Solid Edge part; units mm, degrees
sketch "Sketch1" plane through (0, 0, 0) normal (0, 0, 1) x (1, 0, 0)
  arc A0 (-2.2, 0) -> (-0.6464, 2.8) centre (1.1, 0) cw
  line L0 (-0.6464, 2.8) -> (0, 2.8)
  line L1 (0, 2.8) -> (0, 1.55)
  arc A1 (0, 1.55) -> (0.1, 1.45) centre (0.1, 1.55) ccw
  line L2 (0.1, 1.45) -> (3.9885, 1.45)
  line L3 (3.9885, 1.45) -> (6.5, 0)
  line L4 (6.5, 0) -> (-2.2, 0)
revolve "RevolvedProtrusion1" add sketch "Sketch1" angle 360 about axis through (6.5, 0, 0) along (-1, 0, 0)
sketch "Sketch2" plane through (-2.2, 0, 0) normal (1, 0, 0) x (0, 1, 0)
  line L0 (0.2375, 0.95) -> (-0.2375, 0.95)
  line L1 (-0.2375, 0.95) -> (-0.66, 0.66)
  line L2 (-0.66, 0.66) -> (-0.95, 0.2375)
  line L3 (-0.95, 0.2375) -> (-0.95, -0.2375)
  line L4 (-0.95, -0.2375) -> (-0.66, -0.66)
  line L5 (-0.66, -0.66) -> (-0.2375, -0.95)
  line L6 (-0.2375, -0.95) -> (0.2375, -0.95)
  line L7 (0.2375, -0.95) -> (0.66, -0.66)
  line L8 (0.66, -0.66) -> (0.95, -0.2375)
  line L9 (0.95, -0.2375) -> (0.95, 0.2375)
  line L10 (0.95, 0.2375) -> (0.66, 0.66)
  line L11 (0.66, 0.66) -> (0.2375, 0.95)
extrude "ExtrudedCutout_1" cut sketch "Sketch2" along normal blind 0.7333
sketch "Sketch3" plane through (-2.2, 0, 0) normal (1, 0, 0) x (0, 1, 0)
  line L0 (0.1187, 0.475) -> (-0.1187, 0.475)
  line L1 (-0.1187, 0.475) -> (-0.33, 0.33)
  line L2 (-0.33, 0.33) -> (-0.475, 0.1188)
  line L3 (-0.475, 0.1188) -> (-0.475, -0.1187)
  line L4 (-0.475, -0.1187) -> (-0.33, -0.33)
  line L5 (-0.33, -0.33) -> (-0.1187, -0.475)
  line L6 (-0.1187, -0.475) -> (0.1187, -0.475)
  line L7 (0.1187, -0.475) -> (0.33, -0.33)
  line L8 (0.33, -0.33) -> (0.475, -0.1187)
  line L9 (0.475, -0.1187) -> (0.475, 0.1188)
  line L10 (0.475, 0.1188) -> (0.33, 0.33)
  line L11 (0.33, 0.33) -> (0.1187, 0.475)
extrude "ExtrudedCutout_2" cut sketch "Sketch3" along normal blind 0.88
properties part number "bene_inox_212406-2,9X6,5"
Can you work these out from the model? Positions are in its coordinate system, mm. Give positions to 0.01 mm unless a question says otherwise; leave off trailing zeros. Order: outer loops, then holes, each group sorted by start corner. A loop starts at its lowest first (then second) coordinate and runs counter-clockwise, first axis right, second up. Notation, with made-up numbers: M 46,5 L 56,5 A16 ccw 56,35 Z; hole C 77,14 d7. An arc over 180 degrees is marked long. Use one line per item in the form item = value.
Item 1: Will these pins go through, and if not, where does the flat tip stop? pin 1 Ø0.6 at (y, z) = (0, 0) entering from -X; pin 2 Ø1 at (y, z) = (0, 1.5) entering from -X; pin 3 Ø3 at (x, z) = (4, 0) entering from -Y.
Values follow:
pin_1 = -1.32
pin_2 = -2.04
pin_3 = -1.45
Item 2: If I drill on line 1 along Z through (x, y) = (4.25, -0.05); line 2 along X through (y, z) = (-1.75, -1.85); line 3 along X through (y, z) = (-1.5, -2.3), over which ranges is the centre line in solid material (lowest first)? Write a range as [from, to].
Values follow:
line_1 = [-1.3, 1.3]
line_2 = [-1, 0]
line_3 = [-0.73, 0]
Item 3: Thinking about a two-plate mould opening in Z: for faces 1 (the flat face through (-1.32, 0, 0)), 2 (the flat face through (0, 1.21, 1.21)), 3 (the cylindrical face through (2.07, -1.45, 0.06)), which applies, pulls with the +Z half, pulls with the -Z half, needs draft (parallel to the pull), parting line crosses it, or undercut?
Values follow:
face_1 = undercut
face_2 = needs draft
face_3 = parting line crosses it
Item 4: If we section it at D-D, the plane x = 5: Write out the boundary of the cut face in (y, z).
Values follow:
outline = C 0,0 d1.73
Item 5: If we section it at C-C, the plane y = -2.2: Write out the boundary of the cut face in (x, z).
Values follow:
outline = M -0.65,-1.73 L 0,-1.73 L 0,1.73 L -0.65,1.73 A2.46 ccw Z
Item 6: If we section it at B-B, the plane z = -1.85: Write out the boundary of the cut face in (x, y).
Values follow:
outline = M -0.65,-2.1 L 0,-2.1 L 0,2.1 L -0.65,2.1 A2.73 ccw Z
Item 7: If we section it at A-A, the plane x = 0.25: Write out the boundary of the cut face in (y, z).
Values follow:
outline = C 0,0 d2.9
